Drawing for the job (mm, zero at the part's lowest x, y, z). A direction names the side the tool comes from. Give positions to 0.01 mm unless a question says otherwise; leave off trailing zeros. Order: outer loops, then holes, each group sorted by start corner. A loop starts at its lowest first (then second) coordinate and runs counter-clockwise, first axis right, second up. Notation, with made-up numbers: (52, -13) -> (95, -13) arc R14 ccw to (95, 7) -> close; hole circle Ø1 at (54, 18). An arc over 180 degrees is marked (long way). One line per item, written item: value. Start each with the question number.
(1) Saw through at C-C on z = 1.5. Give the cut face in (x, y) (1 decimal).
(2) Saw through at B-B on y = 25. Give the cut face in (x, z), plus the area to 3 significant figures.
(3) Saw through at D-D on y = 15.5. Count the separate pieces of the cut face and the enclosed holes in it.
(4) Probe line 1 (Y direction, x = 25, z = 7); line 2 (X direction, y = 15.5, z = 7) (1 decimal); line 3 (Y direction, x = 9, z = 6.25). List the from-to ranges inside material, lowest first.
(5) Saw through at A-A on x = 25. Give the cut face in (y, z), plus the area to 3 significant figures.
(6) Pin check, flat tips, straight feed: pin 1 (3 mm diameter, centred on x = 32.5, z = 3, fed in from -Y); pin 2 (6 mm diameter, centred on y = 30, z = 7.5, fed in from +X); pin 3 (2 mm diameter, centred on x = 26, y = 45, fed in from +Z). Stop position of each tip, or through.
(7) Which spindle directions (+Z, -Z, +X, -X, +Y, -Y) get a long thin tool onto all of the face, cutting with end or side? Do the marked faces 4 and 5. Say none if no direction does.
(8) Two-plate mould, pull along Y, no slides. Class the marked faces 1, 2 and 3: +Y half, -Y half, draft (parallel to the pull), parting line (faces both ways), or undercut.
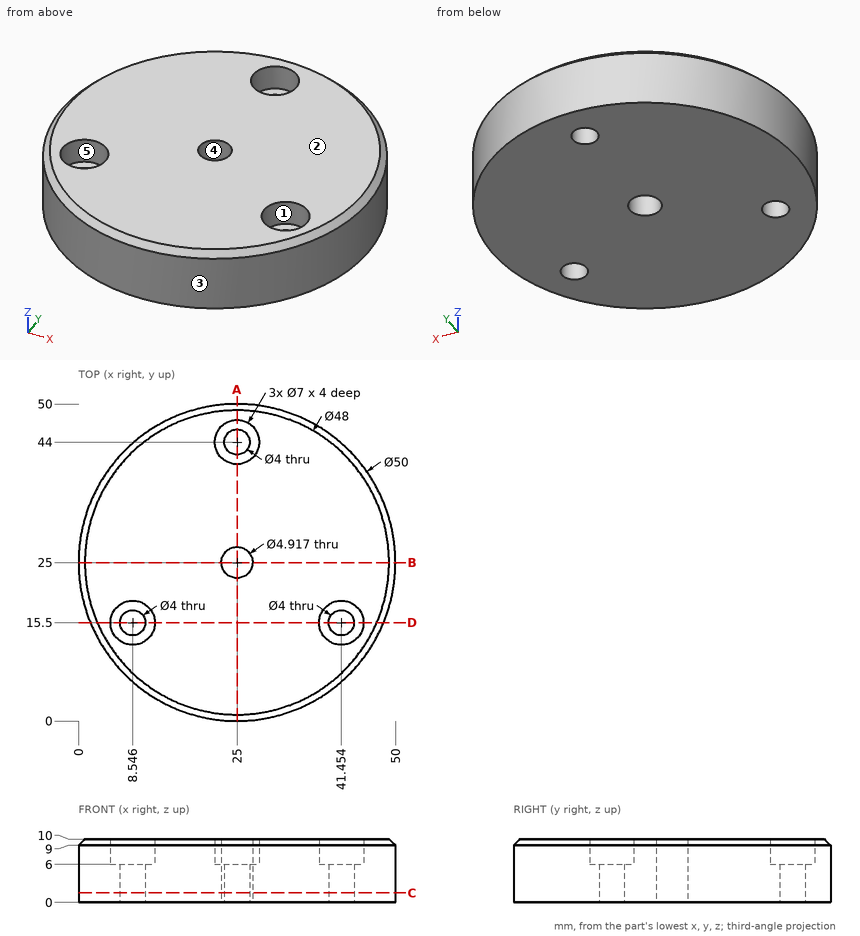
Results below:
1. outline: circle Ø50 at (25, 25); hole circle Ø4 at (8.5, 15.5); hole circle Ø4.9 at (25, 25); hole circle Ø4 at (25, 44); hole circle Ø4 at (41.5, 15.5)
2. outline: (0, 0) -> (22.54, 0) -> (22.54, 10) -> (1, 10) -> (0, 9) -> close; (27.46, 0) -> (50, 0) -> (50, 9) -> (49, 10) -> (27.46, 10) -> close
2. area: 450 mm²
3. separate pieces: 3
3. enclosed holes: 0
4. line 1: y = 0 to 22.54, 27.46 to 40.5, 47.5 to 50
4. line 2: x = 1.9 to 5, 12 to 38, 45 to 48.1
4. line 3: y = 5.79 to 12.03, 18.97 to 44.21
5. outline: (0, 0) -> (22.54, 0) -> (22.54, 10) -> (1, 10) -> (0, 9) -> close; (27.46, 0) -> (42, 0) -> (42, 6) -> (40.5, 6) -> (40.5, 10) -> (27.46, 10) -> close; (46, 0) -> (50, 0) -> (50, 9) -> (49, 10) -> (47.5, 10) -> (47.5, 6) -> (46, 6) -> close
5. area: 398 mm²
6. pin 1: stops at y = 0.73
6. pin 2: stops at x = 49.92
6. pin 3: stops at z = 6
7. face 4: +Z, -Z
7. face 5: +Z
8. face 1: undercut
8. face 2: draft
8. face 3: parting line
